```python
from build123d import *

# Parameters (mm, degrees)
SKETCH1_W                        = 15
SKETCH1_H                        = 6
MAIN_BODY_EXT_DEPTH              = 8.3
EMISSION_PATH_EXT_DEPTH          = 9
SKETCH3_R                        = 1.25
EMISSION_AND_GRIN_CUT_DEPTH      = 20.092931
SKETCH4_R                        = 1
DRUM_LENS_CUT_DEPTH              = 13
SKETCH41_R                       = 1
ADDTL_LIGHT_SOURCE_DEPTH         = 5
SKETCH5_W                        = 15
SKETCH5_H                        = 7.3
FILTERCOVER_CUT1_DEPTH           = 1
TOP_LED_SCREW_W                  = 3.06
TOP_LED_SCREW_H                  = 2
BOSS_EXTRUDE1_DEPTH              = 1
FILTERSET_CUT2_DEPTH             = 4
SKETCH10_R                       = 2.5
EMISSION_LENS_CUT_DEPTH          = 8.5
SKETCH15_R                       = 0.795
MAGNETS_CUT_DEPTH                = 0.9
SCREW_HOLES_CUT_DEPTH            = 20.507434
SCREW_HOLES_CUT_DEPTH_BACK       = 2.5
SKETCH18_R                       = 0.375
EXTERNAL_FILLET_1_R              = 1.5
VERTICAL_PATH_CUT_DEPTH          = 14.011149
VERTICAL_PATH_CUT_DEPTH_BACK     = 4
SKETCH28_R                       = 1.5
CUT_EXTRUDE_ORIGINAL_LIGHT_DEPTH = 0.7
CUT_EXTRUDE_ADDTL_LIGHT_DEPTH    = 0.7
SKETCH29_R                       = 0.375
SIDE_LED_SCREW_DEPTH             = 2.5
SKETCH32_W                       = 2
SKETCH32_H                       = 2.36
SIDE_WIRE_SLOT_CUT_DEPTH         = 0.7
SKETCH45_W                       = 2.36
SKETCH45_H                       = 2
TOP_LED_SLOT_DEPTH               = 0.7
CUT_EXTRUDE16_DEPTH              = 9
CUT_EXTRUDE17_REACH              = 13.945
SKETCH37_R                       = 2
SKETCH51_R                       = 0.375
TOP_LE_SCREW_DEPTH               = 2.1
CUT_EXTRUDE20_DEPTH              = 2


with BuildPart() as part:
    # Sketch1 → Main Body Ext (new body)
    with BuildSketch(Plane(origin=(0, 0, 0), x_dir=(1, 0, 0), z_dir=(0, 1, 0))):
        Rectangle(SKETCH1_W, SKETCH1_H)
    extrude(amount=MAIN_BODY_EXT_DEPTH)

    # Sketch8 → Emission Path Ext (add)
    with BuildSketch(Plane(origin=(0, 8.3, 0), x_dir=(1, 0, 0), z_dir=(0, 1, 0))):
        Polygon((-2.75, 3), (-1.5, 1.75), (-1.5, -3), (-7.5, -3), (-7.5, 3), align=None)
    extrude(amount=EMISSION_PATH_EXT_DEPTH)

    # Sketch3 → Emission and Grin Cut (cut, through all)
    with BuildSketch(Plane.XZ):
        with Locations(Location((-4.5, 0, 0), (0, 0, 270))):
            Circle(SKETCH3_R)
    extrude(amount=-EMISSION_AND_GRIN_CUT_DEPTH, mode=Mode.SUBTRACT)

    # Sketch4 → Drum Lens Cut (cut)
    with BuildSketch(Plane(origin=(7.5, 0, 0), x_dir=(0, 0, -1), z_dir=(1, 0, 0))):
        with Locations((0, 3)):
            Circle(SKETCH4_R)
    extrude(amount=-DRUM_LENS_CUT_DEPTH, mode=Mode.SUBTRACT)

    # Sketch41 → Addtl Light Source (cut)
    with BuildSketch(Plane(origin=(0, 8.3, 0), x_dir=(1, 0, 0), z_dir=(0, 1, 0))):
        with Locations(Location((1.5, 0, 0), (0, 0, 270))):
            Circle(SKETCH41_R)
    extrude(amount=-ADDTL_LIGHT_SOURCE_DEPTH, mode=Mode.SUBTRACT)

    # Sketch5 → FilterCover Cut1 (cut)
    with BuildSketch(Plane.XY.offset(3)):
        with Locations((0, 4.65)):
            Rectangle(SKETCH5_W, SKETCH5_H)
    extrude(amount=-FILTERCOVER_CUT1_DEPTH, mode=Mode.SUBTRACT)

    # Top-LED-Screw → Boss-Extrude1 (add)
    with BuildSketch(Plane.XY.offset(2)):
        with Locations((5.97, 7.3)):
            Rectangle(TOP_LED_SCREW_W, TOP_LED_SCREW_H)
    extrude(amount=BOSS_EXTRUDE1_DEPTH)

    # Sketch6 → FilterSet Cut2 (cut)
    with BuildSketch(Plane.XY.offset(2)):
        with BuildLine():
            Line((5.3, 4.5), (5.3, 1.8))
            ThreePointArc((5.3, 1.8), (5.7, 1.4), (5.3, 1))
            Line((5.3, 1), (4.1, 1))
            ThreePointArc((4.1, 1), (3.7, 1.4), (4.1, 1.8))
            Line((4.1, 1.8), (4.1, 4.5))
            ThreePointArc((4.1, 4.5), (4.7, 5.1), (5.3, 4.5))
        make_face()
        with BuildLine():
            Line((-6.9, 7.9), (-6.9, 7.5))
            ThreePointArc((-6.9, 7.5), (-6.782843, 7.217157), (-6.5, 7.1))
            Line((-6.5, 7.1), (-2.5, 7.1))
            ThreePointArc((-2.5, 7.1), (-2.217157, 7.217157), (-2.1, 7.5))
            Line((-2.1, 7.5), (-2.1, 7.9))
            ThreePointArc((-2.1, 7.9), (-2.217157, 8.182843), (-2.5, 8.3))
            Line((-2.5, 8.3), (-6.5, 8.3))
            ThreePointArc((-6.5, 8.3), (-6.782843, 8.182843), (-6.9, 7.9))
        make_face()
        with BuildLine():
            Line((-2.605887, 6.591169), (-6.848528, 2.348528))
            ThreePointArc((-6.848528, 2.348528), (-6.848528, 1.5), (-6, 1.5))
            Line((-6, 1.5), (-1.757359, 5.742641))
            ThreePointArc((-1.757359, 5.742641), (-1.757359, 6.591169), (-2.605887, 6.591169))
        make_face()
        with BuildLine():
            Line((3.112092, 6.591169), (-1.130548, 2.348528))
            ThreePointArc((-1.130548, 2.348528), (-1.130548, 1.5), (-0.28202, 1.5))
            Line((-0.28202, 1.5), (3.96062, 5.742641))
            ThreePointArc((3.96062, 5.742641), (3.96062, 6.591169), (3.112092, 6.591169))
        make_face()
    extrude(amount=-FILTERSET_CUT2_DEPTH, mode=Mode.SUBTRACT)

    # Sketch10 → Emission Lens Cut (cut)
    with BuildSketch(Plane(origin=(0, 17.3, 0), x_dir=(1, 0, 0), z_dir=(0, 1, 0))):
        with Locations(Location((-4.5, 0, 0), (0, 0, 270))):
            Circle(SKETCH10_R)
    extrude(amount=-EMISSION_LENS_CUT_DEPTH, mode=Mode.SUBTRACT)

    # Sketch15 → Magnets Cut (cut)
    with BuildSketch(Plane.XZ):
        with Locations(Location((-6.25, -1.875, 0), (0, 0, 270))):
            Circle(SKETCH15_R)
        with Locations(Location((-6.25, 1.875, 0), (0, 0, 270))):
            Circle(SKETCH15_R)
        with Locations(Location((-1.5, 0, 0), (0, 0, 270))):
            Circle(SKETCH15_R)
    extrude(amount=-MAGNETS_CUT_DEPTH, mode=Mode.SUBTRACT)

    # Sketch18 → Screw Holes Cut (cut, two sides: drawn at the far end of the back side and taken through both)
    with BuildSketch(Plane.XY.offset(2).offset(-SCREW_HOLES_CUT_DEPTH_BACK)):
        with Locations(Location((-6.5, 4, 0), (0, 0, 180))):
            Circle(SKETCH18_R)
        with Locations(Location((6, 5.8, 0), (0, 0, 180))):
            Circle(SKETCH18_R)
        with Locations((0.25, 1)):
            Circle(SKETCH18_R)
    extrude(amount=SCREW_HOLES_CUT_DEPTH + SCREW_HOLES_CUT_DEPTH_BACK, mode=Mode.SUBTRACT)

    # External Fillet 1
    # the kernel refuses this fillet: 1.5 mm, written as the material it takes off along each edge
    with BuildSketch(Plane(origin=(-7.5, -3.75, -3), x_dir=(1, 0, 0), z_dir=(0, 1, 0))) as external_fillet_1_piece_1:
        with BuildLine():
            CenterArc((EXTERNAL_FILLET_1_R, -EXTERNAL_FILLET_1_R), EXTERNAL_FILLET_1_R, 90, 90)
            Line((0, -EXTERNAL_FILLET_1_R), (0, 0))
            Line((0, 0), (EXTERNAL_FILLET_1_R, 0))
        make_face()
    extrude(amount=24.8, mode=Mode.SUBTRACT)
    with BuildSketch(Plane(origin=(-1.5, 8.3, 3), x_dir=(0, 0, -1), z_dir=(0, 1, 0))) as external_fillet_1_piece_2:
        with BuildLine():
            CenterArc((EXTERNAL_FILLET_1_R, EXTERNAL_FILLET_1_R), EXTERNAL_FILLET_1_R, 180, 90)
            Line((0, EXTERNAL_FILLET_1_R), (0, 0))
            Line((0, 0), (EXTERNAL_FILLET_1_R, 0))
        make_face()
    extrude(amount=12.75, mode=Mode.SUBTRACT)

    # Sketch28 → Vertical-Path-Cut (cut, two sides: drawn at the far end of the back side and taken through both)
    with BuildSketch(Plane(origin=(0, 7.1, 0), x_dir=(1, 0, 0), z_dir=(0, 1, 0)).offset(-VERTICAL_PATH_CUT_DEPTH_BACK)):
        with Locations(Location((-4.5, 0, 0), (0, 0, 180))):
            Circle(SKETCH28_R)
    extrude(amount=VERTICAL_PATH_CUT_DEPTH + VERTICAL_PATH_CUT_DEPTH_BACK, mode=Mode.SUBTRACT)

    # Sketch12 → Cut-Extrude Original Light (cut)
    with BuildSketch(Plane(origin=(7.5, 0, 0), x_dir=(0, 0, -1), z_dir=(1, 0, 0))):
        with BuildLine():
            Line((1.6, 5.94), (-1.6, 5.94))
            Line((-1.6, 5.94), (-2, 5.94))
            Line((-2, 5.94), (-2, 1.33))
            Line((-2, 1.33), (1.6, 1.33))
            ThreePointArc((1.6, 1.33), (1.882843, 1.447157), (2, 1.73))
            Line((2, 1.73), (2, 5.54))
            ThreePointArc((2, 5.54), (1.882843, 5.822843), (1.6, 5.94))
        make_face()
    extrude(amount=-CUT_EXTRUDE_ORIGINAL_LIGHT_DEPTH, mode=Mode.SUBTRACT)

    # Sketch44 → Cut-Extrude Addtl Light (cut)
    with BuildSketch(Plane(origin=(0, 8.3, 0), x_dir=(1, 0, 0), z_dir=(0, 1, 0))):
        with BuildLine():
            Line((-0.17, -2), (4.44, -2))
            Line((4.44, -2), (4.44, 1.6))
            ThreePointArc((4.44, 1.6), (4.322843, 1.882843), (4.04, 2))
            Line((4.04, 2), (0.23, 2))
            ThreePointArc((0.23, 2), (-0.052843, 1.882843), (-0.17, 1.6))
            Line((-0.17, 1.6), (-0.17, -2))
        make_face()
    extrude(amount=-CUT_EXTRUDE_ADDTL_LIGHT_DEPTH, mode=Mode.SUBTRACT)

    # Sketch29 → Side-LED-Screw (cut)
    with BuildSketch(Plane(origin=(7.5, 0, 0), x_dir=(0, 0, -1), z_dir=(1, 0, 0))):
        with Locations((2, 6.5)):
            Circle(SKETCH29_R)
    extrude(amount=-SIDE_LED_SCREW_DEPTH, mode=Mode.SUBTRACT)

    # Sketch32 → Side-Wire-Slot-Cut (cut)
    with BuildSketch(Plane(origin=(7.5, 0, 0), x_dir=(0, 0, -1), z_dir=(1, 0, 0))):
        with Locations((0, 7.12)):
            Rectangle(SKETCH32_W, SKETCH32_H)
    extrude(amount=-SIDE_WIRE_SLOT_CUT_DEPTH, mode=Mode.SUBTRACT)

    # Sketch45 → Top-LED-slot (cut)
    with BuildSketch(Plane(origin=(0, 8.3, 0), x_dir=(1, 0, 0), z_dir=(0, 1, 0))):
        with Locations((5.62, 0)):
            Rectangle(SKETCH45_W, SKETCH45_H)
    extrude(amount=-TOP_LED_SLOT_DEPTH, mode=Mode.SUBTRACT)

    # Sketch33 → Side-BallLens_Cut (revolve, cut)
    with BuildSketch(Plane.XY, mode=Mode.PRIVATE) as side_balllens_cut_sk:
        with BuildLine():
            Line((6.8, 3), (5.3, 3))
            ThreePointArc((5.3, 3), (5.73934, 4.06066), (6.8, 4.5))
            Line((6.8, 4.5), (6.8, 3))
        make_face()
    revolve(side_balllens_cut_sk.sketch.rotate(Axis((6.8, 3, 0), (-1, 0, 0)), 84.26086), axis=Axis((6.8, 3, 0), (-1, 0, 0)), mode=Mode.SUBTRACT)

    # Sketch47 → Top-BallLens_Cut (revolve, cut)
    with BuildSketch(Plane(origin=(1.5, 0, 0), x_dir=(0, 0, -1), z_dir=(1, 0, 0))):
        with BuildLine():
            Line((-1.5, 7.6), (0, 7.6))
            Line((0, 7.6), (0, 6.137287))
            ThreePointArc((0, 6.137287), (-1.04756, 6.563498), (-1.5, 7.6))
        make_face()
    revolve(axis=Axis((1.5, 7.6, 0), (0, -1, 0)), mode=Mode.SUBTRACT)

    # Sketch36 → Cut-Extrude16 (cut)
    with BuildSketch(Plane(origin=(0, 17.3, 0), x_dir=(1, 0, 0), z_dir=(0, 1, 0))):
        with BuildLine():
            Line((-7.5, -1.5), (-7.5, -3))
            Line((-7.5, -3), (-6, -3))
            ThreePointArc((-6, -3), (-7.06066, -2.56066), (-7.5, -1.5))
        make_face()
    extrude(amount=-CUT_EXTRUDE16_DEPTH, mode=Mode.SUBTRACT)

    # Sketch37 → Cut-Extrude17 (cut, up to next)
    with BuildSketch(Plane(origin=(0, 8.8, 0), x_dir=(1, 0, 0), z_dir=(0, 1, 0)), mode=Mode.PRIVATE) as cut_extrude17_sk1:
        with Locations(Location((-4.5, 0, 0), (0, 0, 180))):
            Circle(SKETCH37_R)
    cut_extrude17_tool1 = extrude(cut_extrude17_sk1.sketch, amount=-CUT_EXTRUDE17_REACH, mode=Mode.PRIVATE) & part.part
    add(cut_extrude17_tool1.solids().sort_by_distance((-4.5, 8.8, 0))[0], mode=Mode.SUBTRACT)

    # Sketch51 → Top-LE-Screw (cut)
    with BuildSketch(Plane(origin=(0, 8.3, 0), x_dir=(1, 0, 0), z_dir=(0, 1, 0))):
        with Locations(Location((5, -2, 0), (0, 0, 270))):
            Circle(SKETCH51_R)
    extrude(amount=-TOP_LE_SCREW_DEPTH, mode=Mode.SUBTRACT)

    # Notch → Cut-Extrude20 (cut)
    with BuildSketch(Plane.XZ):
        Polygon((3.181665, -1.6476), (1.6516, -1.6476), (1.6516, -3), (5.210265, -3), align=None)
        Polygon((1.6516, -3), (1.6516, -1.6476), (0.75, -3), align=None)
    extrude(amount=-CUT_EXTRUDE20_DEPTH, mode=Mode.SUBTRACT)


solid = part.part
```
Design review of the part built by this model. Coordinates are the model's own, in mm. A direction names the side the tool comes from. Coordinates: 2 decimals unless noted, no trailing zeros. Write each loop counter-clockwise with the first axis right and the second up, starting at its lowest first coordinate (ties: lowest second). Pieces come first, ordered by that corner, then holes. Notation, with made-up numbers: M 35,-19.5 L 49,-19.5 A3 cw 49,-14.5 Z; hole C 41,-23.75 d1. An arc over 180 degrees is marked long. Answer as a JSON object with one key per item and string values.
Item 1: Add section C-C, the plane y = 2.75. State how many separate pieces and enclosed holes the cut face has, and give its area (3 significant figures).
Outcome:
{"separate pieces": "4", "enclosed holes": "0", "area": "35.4 mm²"}
Item 2: Machinability: for faces 5 (the flat face through (1.21, 0.99, -2.31)), 6 (the cylindrical face through (-2.502, 8.554, 0.088)), 7 (the flat face through (-6.239, 0.9, 1.886)), which of the approach directions +Z, -Z, +X, -X, +Y, -Y give a long, thin tool a straight path to every point of the face, cutting with its end or side? Answer none if there is none.
Outcome:
{"face 5": "-Z, -Y", "face 6": "+Y", "face 7": "-Y"}
Item 3: Draft analysis for pull direction Y (two halves, no side actions). For faces 1 (the flat face through (-6, 0.9, -2)), 2 (the flat face through (6, 8.3, 2)), 3 (the cylindrical face through (3.7, 1.4, 0)), 4 (the flat face through (4.1, 4, 1)), state which applies: pulls with the +Y half, pulls with the -Y half, needs draft (parallel to the pull), parting line crosses it, or undercut.
Outcome:
{"face 1": "pulls with the -Y half", "face 2": "pulls with the +Y half", "face 3": "undercut", "face 4": "undercut"}
Item 4: Add section A-A, the plane y = 13.75. Give the boundary of the cut face in (x, z).
Outcome:
{"outline": "M -7.5,-1.5 A1.5 ccw -6,-3 L -2.75,-3 L -1.5,-1.75 L -1.5,1.5 A1.5 ccw -3,3 L -6,3 A1.5 ccw -7.5,1.5 Z; hole C -4.5,0 d5"}
Item 5: Insertion check: pin 1 Ø2.5 at (y, z) = (3, 0) entering from +X; pin 2 Ø0.6 at (x, y) = (-4, 7.5) entering from +Z; pin 3 Ø1.5 at (x, z) = (1, 0) entering from +Y. Each pin has a flat end and moves straight along its axis. Give the tip position at first contact, or say it passes through.
Outcome:
{"pin 1": "x = 5.97", "pin 2": "z = -2", "pin 3": "y = 6.81"}
Item 6: Add section B-B, the plane y = 4.75. Give the boundary of the cut face in (x, z), and give its area (3 significant figures).
Outcome:
{"outline": "M -7.5,-1.5 A1.5 ccw -6,-3 L 7.5,-3 L 7.5,-2 L 6.8,-2 L 6.8,2 L 5.25,2 L 5.25,-2 L 4.15,-2 L 4.15,2 L 2.97,2 L 2.97,-2 L 1.27,-2 L 1.27,-0.97 A1 cw 1.27,0.97 L 1.27,2 L -2.75,2 L -2.75,-2 L -4.45,-2 L -4.45,-1.5 A1.5 cw long -4.45,1.5 L -4.45,2 L -7.5,2 Z", "area": "49.0 mm²"}
Item 7: Wall thickness on probe 1 along X at (y, z) = (0.35, 0) (3 decimals); probe 2 along Y at (x, z) = (6.5, 2.35); probe 3 along Y at (x, z) = (-2.75, -0.5): over which ranges is each line inside the solid? List them lowest first.
Outcome:
{"probe 1": "-7.5 to -5.75, -3.25 to -2.295, -0.705 to 7.5", "probe 2": "0 to 1, 6.3 to 8.3", "probe 3": "0 to 2.13, 3.87 to 4.75, 6.45 to 7.1"}
